Input: part model. Units: mm. Frame: model coordinates. Face numbers are marked on the shaded views. Round coordinates to 2 decimals unless told otherwise and drop trailing zeros. Order: outer loops, then holes, each group sorted by start corner. A loop starts at its lowest first (then second) coordinate and runs counter-clockwise, first axis right, second up. Notation, with made-up numbers: (-10, 5) -> (24, 5) arc R14 cw to (24, 17) -> close; hole circle Ø9 at (-30, -27). An arc over 180 degrees is marked (long way). Use a Markdown table: item, result.
from build123d import *

# Parameters (mm, degrees)
EXTRUDE_5_REACH          = 62.717
EXTRUDE_5_START_RADIUS   = 22
EXTRUDE_5_END_RADIUS     = 22
PATTERN_CIRCULAR_2_COUNT = 6
CUT_EXTRUDE_1_DEPTH      = 0.2
FILLET_1_R               = 0.05
CHAMFER_1_SIZE           = 0.3


with BuildPart() as part:
    # 草图1 → 旋转1 (revolve)
    with BuildSketch(Plane.XY, mode=Mode.PRIVATE) as revolve_1_sk:
        with BuildLine():
            Line((-22, 0), (-23.5, 0))
            Line((-23.5, 0), (-23.5, 24.150257739))
            ThreePointArc((-23.5, 24.150257739), (-23.399484522, 24.525386608), (-23.124871131, 24.8))
            Line((-23.124871131, 24.8), (-20.7, 26.2))
            Line((-20.7, 26.2), (-18.5, 26.2))
            Line((-18.5, 26.2), (-18.5, 25.2))
            Line((-18.5, 25.2), (-16.5, 25.2))
            Line((-16.5, 25.2), (-16.5, 24.4))
            Line((-16.5, 24.4), (-22, 24.4))
            Line((-22, 24.4), (-22, 0))
        make_face()
    revolve(revolve_1_sk.sketch.rotate(Axis((0, 0, 0), (0, 1, 0)), 270), axis=Axis((0, 0, 0), (0, 1, 0)))

    # 凸台-拉伸5: from a cylinder face, 62.717 long prism both ways, kept between that surface and its translate by the depth
    extrude_5_start = Plane(origin=(0, 16.4, 0), z_dir=(0, -1, 0)) * Cylinder(EXTRUDE_5_START_RADIUS, 170.434, mode=Mode.PRIVATE)
    extrude_5_end = Plane(origin=(2, 16.4, 0), z_dir=(0, -1, 0)) * Cylinder(EXTRUDE_5_END_RADIUS, 170.434, mode=Mode.PRIVATE)
    # 草图5 → 凸台-拉伸5 (add, from a surface)
    with BuildSketch(Plane.ZY.offset(23.5), mode=Mode.PRIVATE) as extrude_5_sk1:
        Polygon((-0.75, 13.9), (-0.75, 18.9), (0.75, 18.9), (0.75, 13.9), (1.75, 13.9), (1.75, 19.7), (-1.75, 19.7), (-1.75, 13.9), align=None)
    extrude_5_tool1 = extrude(extrude_5_sk1.sketch, amount=EXTRUDE_5_REACH, both=True, mode=Mode.PRIVATE)
    extrude_5 = ((extrude_5_tool1 & extrude_5_start) - extrude_5_end).solids().sort_by_distance((-20.95875, 16.4, -0.817742))[0]
    add(extrude_5)

    # 阵列(圆周)2: 凸台-拉伸5 ×6 about axis
    pattern_circular_2_axis = Axis((0, 0, 0), (0, 1, 0))
    for i in range(1, PATTERN_CIRCULAR_2_COUNT):
        add(extrude_5.rotate(pattern_circular_2_axis, i * 360 / PATTERN_CIRCULAR_2_COUNT))

    # 草图6 → 切除-拉伸1 (cut)
    with BuildSketch(Plane(origin=(0, 26.2, 0), x_dir=(1, 0, 0), z_dir=(0, 1, 0))):
        Polygon((-20.4, 0.468911087), (-18.65, 0), (-20.4, -0.468911087), align=None)
    extrude(amount=-CUT_EXTRUDE_1_DEPTH, mode=Mode.SUBTRACT)

    # 圆角1
    fillet_1_edges = [part.edges().sort_by_distance(p)[0] for p in [
        (-20.4, 26.1, 0.468911087),
        (-20.4, 26.1, -0.468911087),
        (-18.65, 26.1, 0),
    ]]
    fillet(fillet_1_edges, radius=FILLET_1_R)

    # 倒角1
    chamfer_1_edges = [part.edges().sort_by_distance(p)[0] for p in [
        (11.143125149, 13.9, 17.800458913),
        (9.844087043, 13.9, 18.550458913),
        (-9.844087043, 13.9, 18.550458913),
        (-11.143125149, 13.9, 17.800458913),
        (-20.987212193, 13.9, 0.75),
        (-20.987212193, 13.9, -0.75),
        (-11.143125149, 13.9, -17.800458913),
        (-9.844087043, 13.9, -18.550458913),
        (9.844087043, 13.9, -18.550458913),
        (11.143125149, 13.9, -17.800458913),
        (20.987212193, 13.9, -0.75),
        (20.987212193, 13.9, 0.75),
    ]]
    chamfer(chamfer_1_edges, length=CHAMFER_1_SIZE)


solid = part.part
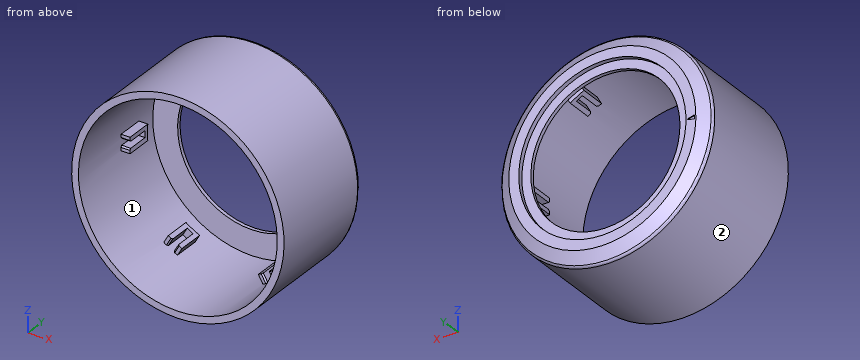
1) Contact query for flat-ended pins moving along their axis: P1, Ø1.5, axis at y = 21.5, z = -13, coming from the -X side; P2, Ø8, axis at y = 13.5, z = 17.5, coming from the -X side; P3, Ø4, axis at x = 10.5, z = -18.5, coming from the +Y side; P4, Ø0.5, axis at x = 9.5, z = -19.5, coming from the -Y side. Output: stop coordinate, or through.
Answer key:
| item | result |
|---|---|
| P1 | stops at x = -20.05 |
| P2 | stops at x = -19.24 |
| P3 | stops at y = 26.2 |
| P4 | stops at y = 13.9 |
2) Cut plane B-B on y = 4.75. Return loops of the section in (x, z), and give its area (3 significant figures).
Answer key:
| item | result |
|---|---|
| outline | circle Ø47 at (0, 0); hole circle Ø44 at (0, 0) |
| area | 214 mm^2 |
3) Draft query along X for the marked faces 1 and 2. Return one class per face: released by +X, released by -X, zero draft, split by the parting line, or undercut.
Answer key:
| item | result |
|---|---|
| face 1 | undercut |
| face 2 | split by the parting line |
4) Cut plane A-A on x = 0. Return loops of the section in (y, z), and give its area (3 significant figures).
Answer key:
| item | result |
|---|---|
| outline | (0, -23.5) -> (24.15, -23.5) arc R0.75 ccw to (24.8, -23.12) -> (26.2, -20.7) -> (26.2, -18.5) -> (25.2, -18.5) -> (25.2, -16.5) -> (24.4, -16.5) -> (24.4, -22) -> (0, -22) -> close; (0, 22) -> (24.4, 22) -> (24.4, 16.5) -> (25.2, 16.5) -> (25.2, 18.5) -> (26.2, 18.5) -> (26.2, 20.7) -> (24.8, 23.12) arc R0.75 ccw to (24.15, 23.5) -> (0, 23.5) -> close |
| area | 89.8 mm^2 |
5) Ray query, probe 1 along X at (y, z) = (18.5, 0); probe 2 along Z at (x, y) = (-0.5, 18.5); probe 3 along X at (y, z) = (23.25, -8). Return the intervals inside material, ascending.
Answer key:
| item | result |
|---|---|
| probe 1 | x = -23.5 to -22, 22 to 23.5 |
| probe 2 | z = -23.49 to -21.99, 21.99 to 23.49 |
| probe 3 | x = -22.1 to -20.49, 20.49 to 22.1 |
